Verification items for the finished model (mm, model axes). A direction names the side the tool comes from. Coordinates: 2 decimals unless noted, no trailing zeros. Write each loop counter-clockwise with the first axis right and the second up, starting at its lowest first coordinate (ties: lowest second). Pieces come first, ordered by that corner, then holes. Notation, with made-up numbers: (36, 72) - (50, 72) arc R7 ccw to (50, 77) - close; hole circle Ø9 at (52.5, 9). An arc over 180 degrees is marked (long way). Use CSV: the item, a comma, the result in double quotes. Start each with the question number.
```python
from build123d import *

# Parameters (mm, degrees)
F1_DEPTH = 2.5
F3_DEPTH = 1.5
F5_DEPTH = 3
F7_DEPTH = 7
F8_SIZE  = 1.25
F9_R     = 1


with BuildPart() as f1:
    # F0 (on Front) → F1 (new body)
    with BuildSketch(Plane.XZ):
        with BuildLine():
            ThreePointArc((17.8, 0), (0, -17.8), (-17.8, 0))
            Line((-17.8, 0), (-21.4427768058, 3.6427768058))
            ThreePointArc((-21.4427768058, 3.6427768058), (0, -21.75), (21.4427768058, 3.6427768058))
            Line((21.4427768058, 3.6427768058), (17.8, 0))
        make_face()
    extrude(amount=F1_DEPTH)

    # F2 (on face) → F3 (join)
    with BuildSketch(Plane.XZ.offset(2.5)):
        with BuildLine():
            ThreePointArc((-21.4427768058, 3.6427768058), (-1.8278545448, -21.6730581082), (21.75, 0))
            ThreePointArc((21.75, 0), (21.6730581082, 1.8278545448), (21.4427768058, 3.6427768058))
            Line((21.4427768058, 3.6427768058), (19.8904504002, 2.0904504002))
            ThreePointArc((19.8904504002, 2.0904504002), (19.9725938226, 1.0466594468), (20, 0))
            ThreePointArc((20, 0), (-1.0466594468, -19.9725938226), (-19.8904504002, 2.0904504002))
            Line((-19.8904504002, 2.0904504002), (-21.4427768058, 3.6427768058))
        make_face()
    extrude(amount=F3_DEPTH)

    # F4 (on face) → F5 (join)
    with BuildSketch(Plane.XZ.offset(4)):
        with BuildLine():
            ThreePointArc((-21.4427768058, 3.6427768058), (-1.8278545448, -21.6730581082), (21.75, 0))
            ThreePointArc((21.75, 0), (21.6730581082, 1.8278545448), (21.4427768058, 3.6427768058))
            Line((21.4427768058, 3.6427768058), (19.8904504002, 2.0904504002))
            ThreePointArc((19.8904504002, 2.0904504002), (0, -20), (-19.8904504002, 2.0904504002))
            Line((-19.8904504002, 2.0904504002), (-21.4427768058, 3.6427768058))
        make_face()
        with BuildLine():
            Line((19.8904504002, 2.0904504002), (21.4427768058, 3.6427768058))
            ThreePointArc((21.4427768058, 3.6427768058), (0, 21.75), (-21.4427768058, 3.6427768058))
            Line((-21.4427768058, 3.6427768058), (-19.8904504002, 2.0904504002))
            ThreePointArc((-19.8904504002, 2.0904504002), (0, -20), (19.8904504002, 2.0904504002))
        make_face()
    extrude(amount=F5_DEPTH)

    # F6 (on face) → F7 (join, through all)
    with BuildSketch(Plane.XZ.offset(7)):
        with BuildLine():
            ThreePointArc((-6.4e-09, -21.75), (-15.3795724931, -15.3795724885), (-21.75, 0))
            Line((-21.75, 0), (-21.75, -21.75))
            Line((-21.75, -21.75), (-6.4e-09, -21.75))
        make_face()
        with BuildLine():
            Line((21.75, -21.75), (21.75, 0))
            ThreePointArc((21.75, 0), (15.3795724885, -15.3795724931), (-6.4e-09, -21.75))
            Line((-6.4e-09, -21.75), (21.75, -21.75))
        make_face()
    extrude(amount=-F7_DEPTH)

    # F8
    f8_edges = [f1.edges().sort_by_distance(p)[0] for p in [
        (0, -4, 21.75),
        (18.845225, -2.5, 1.045225),
        (0, -2.5, -17.8),
        (-18.845225, -2.5, 1.045225),
    ]]
    chamfer(f8_edges, length=F8_SIZE)

    # F9
    f9_edges = [f1.edges().sort_by_distance(p)[0] for p in [
        (21.75, 0, -10.875),
        (-21.75, 0, -10.875),
    ]]
    fillet(f9_edges, radius=F9_R)


solid = f1.part
```
Q1. Cross-section at A-A (x = 0). Record the cut outline in (y, z).
Q2. Gauge pin test, flat end, axial feed: pin 1 (10 mm diameter, centred on x = -16.5, z = 11.5, fed in from +Y). Record the tip position at first contact, or that the pin passes through.
Q3. Tool access check on faces 1 (the flat face through (0, -4, 1)), 2 (the cylindrical face through (0.391, -0.616, -17.796)), 3 (the flat face through (-21.75, -4, -11)). Record the directions out of +Z, -Z, +X, -X, +Y, -Y that give a thin tool (end or side, any length) a straight path to the whole face; none if there is none.
Q4. Scan lines: line 1 along Y through (x, z) = (8, 4); line 2 along X through (y, z) = (-3.5, -8); line 3 along X through (y, z) = (-1.75, -16). Record each from-to range of solid material in increasing order. Write a range as from..to.
Q5. Release check for a two-part mould opening along Y. For faces 4 (the flat face through (0, -4, -21.75)), 5 (the flat face through (-3, -2.5, -19)), 6 (the cylindrical face through (21.465, -0.301, -10.723)) record: released by +Y, released by -Y, zero draft, split by the parting line, or undercut.
Reply:
1,outline,"(-7, -21.75) - (0, -21.75) - (0, -17.8) - (-1.25, -17.8) - (-2.5, -19.05) - (-2.5, -20) - (-4, -20) - (-4, 20.5) - (-5.25, 21.75) - (-7, 21.75) - close"
2,pin 1,"y = -4"
3,face 1,"+Z"
3,face 2,"+Z, +Y"
3,face 3,"+Z, -Z, -X, +Y, -Y"
4,line 1,"-7..-4"
4,line 2,"-21.75..-18.33, 18.33..21.75"
4,line 3,"-21.75..-8.88, 8.88..21.75"
5,face 4,"zero draft"
5,face 5,"undercut"
5,face 6,"released by +Y"
